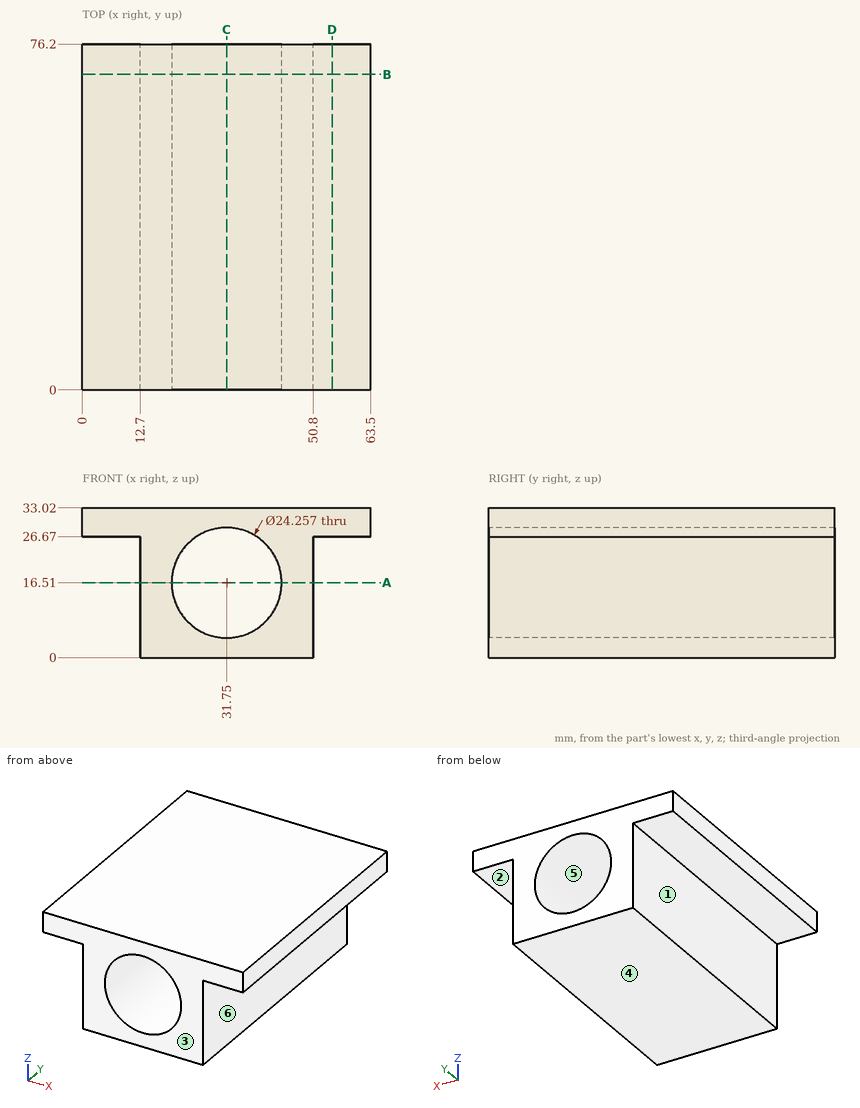
Could you check a few things on this drawing? It's one solid part, dimensions in mm from its lowest x, y, z. A direction names the side the tool comes from. Coordinates: 2 decimals unless noted, no trailing zeros. Order: outer loops, then holes, each group sorted by start corner. A loop starts at its lowest first (then second) coordinate and runs counter-clockwise, first axis right, second up.
1) I need wall thicknesses on line 1 (X direction, y = 39, z = 16); line 2 (Z direction, x = 31.75, y = 33.5); line 3 (Z direction, x = 51.5, y = 8). Which ranges of each line are inside material? Lowest first, please.
2) We'd pull the mould along X, two halves only. Please class the marked faces 4, 5 and 6: +X half, -X half, draft (parallel to the pull), parting line (faces both ways), or undercut.
3) Imagine slicing it at A-A on z = 16.51. List the corners of the cut face in (x, y) for me, and give its area (3 significant figures).
4) Will these pins go through, and if not, where does the flat tip stop? pin 1 (2 mm diameter, centred on y = 44.5, z = 5, fed in from +X); pin 2 (2 mm diameter, centred on y = 21, z = 4.5, fed in from -X); pin 3 (8 mm diameter, centred on x = 13, y = 16, fed in from -Z); pin 4 (10 mm diameter, centred on x = 5.5, y = 39.5, fed in from -Z).
5) Imagine slicing it at B-B on y = 69.5. List the corners of the cut face in (x, z) for me, and give its area (3 significant figures).
6) Imagine slicing it at C-C on x = 31.75. List the corners of the cut face in (y, z) for me, and give its area (3 significant figures).
7) Which directions (+Z, -Z, +X, -X, +Y, -Y) give clear straight access to the entire face, cutting with the end or side of a thin tool? Please do the marked faces 1, 2 and 3.
8) Imagine slicing it at D-D on x = 55. List the corners of the cut face in (y, z) for me.
Response values:
1. line 1: x = 12.7 to 19.63, 43.87 to 50.8
1. line 2: z = 0 to 4.38, 28.64 to 33.02
1. line 3: z = 26.67 to 33.02
2. face 4: draft
2. face 5: undercut
2. face 6: +X half
3. outline: (12.7, 0) - (19.62, 0) - (19.62, 76.2) - (12.7, 76.2) - close; (43.88, 0) - (50.8, 0) - (50.8, 76.2) - (43.88, 76.2) - close
3. area: 1,050 mm2
4. pin 1: stops at x = 50.8
4. pin 2: stops at x = 12.7
4. pin 3: stops at z = 0
4. pin 4: stops at z = 26.67
5. outline: (0, 26.67) - (12.7, 26.67) - (12.7, 0) - (50.8, 0) - (50.8, 26.67) - (63.5, 26.67) - (63.5, 33.02) - (0, 33.02) - close; hole circle Ø24.26 at (31.75, 16.51)
5. area: 957 mm2
6. outline: (0, 0) - (76.2, 0) - (76.2, 4.38) - (0, 4.38) - close; (0, 28.64) - (76.2, 28.64) - (76.2, 33.02) - (0, 33.02) - close
6. area: 668 mm2
7. face 1: -Z, -X, +Y, -Y
7. face 2: -Z, +X, +Y, -Y
7. face 3: +Z, -Z, +X, -X, -Y
8. outline: (0, 26.67) - (76.2, 26.67) - (76.2, 33.02) - (0, 33.02) - close
